CAD build for the part. Positions are in the model's coordinates, mm. Face numbers are marked on the shaded views. Coordinates: 2 decimals unless noted, no trailing zeros. Loops run counter-clockwise (first coordinate to the right, second up) from the corner with the lowest first, then second, coordinate; pieces in that order, holes last.
1) Saw through at A-A, the plane y = -3. Write the cut outline in (x, z), and give its area (3 significant figures).
2) Pin check, flat tips, straight feed: pin 1 Ø3.5 at (x, y) = (-6.5, -21) entering from +Z; pin 2 Ø8 at (x, y) = (6.5, -19.5) entering from +Z; pin 3 Ø8 at (x, z) = (3.5, -2) entering from -Y; pin 4 Ø5 at (x, z) = (0, -6) entering from +Y. Stop position of each tip, or through.
3) Saw through at C-C, the plane z = 7.5. Write the cut outline in (x, y) (3 decimals).
4) Saw through at B-B, the plane z = 0. Write the cut outline in (x, y) (3 decimals).
5) Two-plate mould, pull along Z, no slides. Class the marked faces 1, 2 and 3: +Z half, -Z half, draft (parallel to the pull), parting line (faces both ways), or undercut.
6) Wall check: line 1 along X through (y, z) = (3.35, 0) (3 decimals); line 2 along Y through (x, z) = (-6.5, -29.65) (3 decimals); line 3 along X through (y, z) = (-9, -31) (3 decimals). Give the ranges that are in metal, low to high.
7) Saw through at D-D, the plane x = 1.25. Write the cut outline in (y, z), and give its area (3 significant figures).
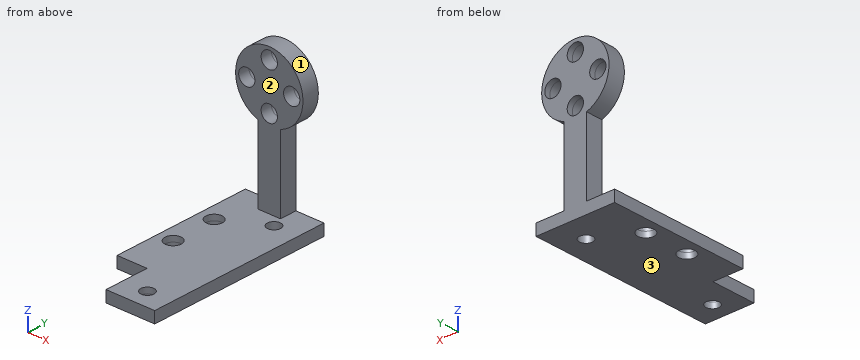
Autodesk Inventor part; units mm, degrees
ref_plane "YZ Plane" through (0, 0, 0) normal (1, 0, 0) x (0, 1, 0)
ref_plane "XZ Plane" through (0, 0, 0) normal (0, 1, 0) x (-1, 0, 0)
ref_plane "XY Plane" through (0, 0, 0) normal (0, 0, 1) x (1, 0, 0)
sketch "Sketch1" plane through (0, 0, 0) normal (0, 1, 0) x (-1, 0, 0)
  arc A0 (3, -8.4853) -> (-3, -8.4853) centre (0, 0) ccw
  circle A1 centre (6, 0) radius 2.175
  circle A2 centre (0, -6) radius 2.175
  circle A3 centre (0, 6) radius 2.175
  circle A4 centre (-6, 0) radius 2.175
  line L0 (-3, -8.4853) -> (-3, -28.4853)
  line L1 (-3, -28.4853) -> (3, -28.4853)
  line L2 (3, -28.4853) -> (3, -8.4853)
  dimension "d0" = 18
  dimension "d1" = 4.35
  dimension "d2" = 6
  dimension "d3" = 4.35
  dimension "d4" = 6
  dimension "d5" = 4.35
  dimension "d6" = 6
  dimension "d7" = 4.35
  dimension "d8" = 6
  dimension "d13" = 6
  dimension "d66" = 20
extrude "Extrusion1" add sketch "Sketch1" along normal blind 3
sketch "Sketch2" plane through (0, 3, 0) normal (0, 1, 0) x (1, 0, 0)
  line L0 (3, 28.4853) -> (-3, 28.4853)
  line L1 (-3, 28.4853) -> (3, 28.4853)
  line L2 (3, 28.4853) -> (3, 29.9853)
  line L3 (3, 29.9853) -> (-3, 29.9853)
  line L4 (-3, 29.9853) -> (-3, 28.4853)
  point P0 (0, 0)
  dimension "d14" = 6
  dimension "d15" = 1.5
extrude "Extrusion2" add sketch "Sketch2" against normal blind 48
sketch "Sketch3" plane through (3, 3, -29.9853) normal (0, 0, -1) x (-1, 0, 0)
  line L0 (0, -3) -> (0, -48)
  line L1 (0, -48) -> (-3.5, -48)
  line L2 (-3.5, -48) -> (-3.5, 0)
  line L3 (-5.175, 0) -> (-0.825, 0)
  line L4 (-3.5, 0) -> (0, 0)
  line L5 (0, 0) -> (0, -48)
  line L6 (0, -48) -> (6, -48)
  line L7 (6.825, 0) -> (11.175, 0)
  line L8 (6, -48) -> (9.5, -48)
  line L9 (9.5, -48) -> (9.5, 0)
  line L10 (9.5, 0) -> (6, 0)
  line L11 (6, 0) -> (6, -48)
  line L12 (9.5, 0) -> (9.5, -48)
  line L13 (-3.5, -48) -> (-7.5, -48)
  line L14 (-7.5, -48) -> (-7.5, 0)
  line L15 (-7.5, 0) -> (-3.5, 0)
  line L16 (-3.5, 0) -> (-3.5, -48)
  line L17 (9.5, -48) -> (13.5, -48)
  line L18 (13.5, -48) -> (13.5, 0)
  line L19 (13.5, 0) -> (9.5, 0)
  line L20 (9.5, 0) -> (9.5, -48)
  point P0 (3, -3)
  dimension "d18" = 3.5
  dimension "d19" = 3.5
  dimension "d43" = 4
  dimension "d44" = 4
extrude "Extrusion3" add sketch "Sketch3" against normal blind 1.5
sketch "Sketch4" plane through (6.5, -45, -29.9853) normal (0, 0, -1) x (-1, 0, 0)
  circle A0 centre (2.5, 5) radius 1.75
  line L0 (-4, 0) -> (17, 0)
  line L1 (17, 0) -> (-4, 0)
  circle A1 centre (2.5, 42) radius 1.75
  line L2 (-2.5, 45) -> (15.5, 45)
  line L3 (-4, 48) -> (-4, 0)
  point P0 (6.5, 45)
  point P1 (0, 0)
  point P2 (21, 0)
  point P3 (0, 48)
  point P4 (3.5, 45)
  point P5 (9.5, 45)
  point P6 (9.5, 0)
  point P7 (3.5, 0)
  point P8 (13, 0)
  dimension "d23" = 3.5
  dimension "d26" = 3.5
  dimension "d28" = 3
  dimension "d45" = 6.5
  dimension "d46" = 6.5
  dimension "d78" = 37
hole "Hole1" at (4, -40, -29.9853) at (4, -3, -29.9853) direction (0, 0, 1) diameter 3.5 depth 8 tip angle 118
sketch "Sketch5" plane through (6.5, -45, -29.9853) normal (0, 0, -1) x (-1, 0, 0)
  line L0 (0.0281, 45) -> (0.0281, 42)
  line L1 (0.0281, 42) -> (0.0281, 30)
  line L2 (0.0281, 30) -> (17, 30)
  line L3 (17, 48) -> (17, 0)
  circle A0 centre (13, 36) radius 2.175
  circle A1 centre (13, 24) radius 2.175
  dimension "d36" = 3
  dimension "d47" = 12
  dimension "d48" = 4.35
  dimension "d49" = 6
  dimension "d50" = 4
  dimension "d51" = 4.35
  dimension "d52" = 6
  dimension "d53" = 4
hole "Hole2" at (-6.5, -21, -29.9853) at (-6.5, -9, -29.9853) direction (0, 0, 1) diameter 4.35 depth 8 tip angle 118
sketch "Sketch6" plane through (10.5, -45, -29.9853) normal (0, 0, -1) x (-1, 0, 0)
  line L0 (0, 0) -> (13, 0)
  line L1 (21, 0) -> (0, 0)
  line L2 (13.5, 48) -> (21, 48)
  line L3 (13, 0) -> (13, 12)
  line L4 (12.675, 45) -> (12.675, 48)
  line L5 (17.25, 24) -> (29.25, 24) construction
  line L6 (21, 12) -> (17.25, 12)
  line L7 (21, 48) -> (21, 0)
  line L8 (21, 12) -> (21, 0)
  line L9 (21, 0) -> (13, 0)
  line L10 (13, 0) -> (13, 12)
  line L11 (13, 12) -> (21, 12)
  point P0 (10.5, 45)
  dimension "d61" = 13
extrude "Extrusion4" cut sketch "Sketch6" against normal through all
sketch "Sketch7" plane through (0, 3, 0) normal (0, 1, 0) x (1, 0, 0)
  line L0 (10.5, 29.9853) -> (-10.5, 29.9853)
  line L1 (-10.5, 29.9853) -> (-10.5, 28.4853)
  line L2 (-10.5, 29.9853) -> (-10.5, 28.4853)
  line L3 (-3, 28.4853) -> (-10.5, 28.4853)
  line L4 (-10.5, 28.4853) -> (-3, 28.4853)
  line L5 (-3, 8.4853) -> (-3, 28.4853)
  line L6 (-3, 28.4853) -> (-3, 8.4853)
  line L7 (10.5, 29.9853) -> (10.5, 28.4853)
  line L8 (-10.5, 29.9853) -> (10.5, 29.9853)
  line L9 (10.5, 29.9853) -> (10.5, 28.4853)
  line L10 (3, 28.4853) -> (3, 8.4853)
  line L11 (10.5, 28.4853) -> (3, 28.4853)
  line L12 (3, 28.4853) -> (3, 8.4853)
  arc A0 (-3, 8.4853) -> (3, 8.4853) centre (0, 0) ccw
  circle A1 centre (0, 6) radius 2.175
  circle A2 centre (-6.0102, 0) radius 2.175
  circle A3 centre (6, 0) radius 2.175
  circle A4 centre (0, -6) radius 2.175
  dimension "d67" = 4.35
  dimension "d68" = 6
  dimension "d69" = 4.35
  dimension "d70" = 6
  dimension "d71" = 4.35
  dimension "d72" = 6
extrude "Extrusion5" add sketch "Sketch7" along normal blind 1.5
sketch "Sketch8" plane through (10.5, -45, -29.9853) normal (0, 0, -1) x (-1, 0, 0)
  line L0 (13, 0) -> (13, 12)
  line L1 (13, -0.1664) -> (13, 12)
  line L2 (13, 12) -> (21, 12)
  line L3 (13, 12) -> (21, 12)
  line L4 (0, 49.5) -> (21, 49.5)
  line L5 (21, 12) -> (21, 49.5)
  line L6 (21, 49.5) -> (0, 49.5)
  line L7 (0, 0) -> (13, 0)
  line L8 (0, 49.5) -> (0, 0)
  line L9 (0, 49.5) -> (0, 0)
  line L10 (0, 0) -> (13, 0)
  circle A0 centre (6.5, 42) radius 1.75
  circle A1 centre (6.5, 42) radius 1.75
  circle A2 centre (17, 24) radius 2.175
  circle A3 centre (17, 24) radius 2.175
  circle A4 centre (17, 36) radius 2.175
  circle A5 centre (17, 36) radius 2.175
  circle A6 centre (6.5, 5) radius 1.75
  circle A7 centre (6.5, 5) radius 1.75
  point P0 (10.5, 45)
  dimension "d75" = 3.5
extrude "Extrusion6" add sketch "Sketch8" along normal blind 1.5
properties part number "leverServoMount"
Data:
1. outline: (-10.5, -31.49) - (2.25, -31.49) - (2.25, -28.49) - (-10.5, -28.49) - close; (5.75, -31.49) - (10.5, -31.49) - (10.5, -28.49) - (5.75, -28.49) - close
1. area: 52.5 mm2
2. pin 1: passes through
2. pin 2: stops at z = -28.49
2. pin 3: stops at y = 0
2. pin 4: stops at y = 4.5
3. outline: (-4.975, 0) - (-1.575, 0) - (-1.575, 4.5) - (-4.975, 4.5) - close; (1.575, 0) - (4.975, 0) - (4.975, 4.5) - (1.575, 4.5) - close
4. outline: (-9, 0) - (-8.175, 0) - (-8.175, 3) - (-8.185, 3) - (-8.185, 4.5) - (-9, 4.5) - close; (-3.835, 3) - (-3.825, 3) - (-3.825, 0) - (3.825, 0) - (3.825, 4.5) - (-3.835, 4.5) - close; (8.175, 0) - (9, 0) - (9, 4.5) - (8.175, 4.5) - close
5. face 1: undercut
5. face 2: draft
5. face 3: -Z half
6. line 1: x = -9 to -8.185, -3.835 to 3.825, 8.175 to 9
6. line 2: y = -33 to -23.175, -18.825 to -11.175, -6.825 to 4.5
6. line 3: x = -10.5 to -8.675, -4.325 to 10.5
7. outline: (-45, -31.49) - (4.5, -31.49) - (4.5, -7.78) - (0, -7.78) - (0, -28.49) - (-45, -28.49) - close; (0, -4.22) - (4.5, -4.22) - (4.5, 4.22) - (0, 4.22) - close; (0, 7.78) - (4.5, 7.78) - (4.5, 8.91) - (0, 8.91) - close
7. area: 285 mm2
